Input: part model. Units: mm. Frame: model coordinates. A direction names the side the tool comes from. Give positions to 0.01 mm unless a question says otherwise; leave off trailing zeros. Loops run counter-clockwise (first coordinate to the right, second up) from the corner with the lowest first, then second, coordinate; pieces in that order, holes last.
from build123d import *

# Parameters (mm, degrees)
SKETCH1_R                       = 6.35
SKETCH1_R_2                     = 3.96875
BOSS_EXTRUDE1_DEPTH             = 7.62
SKETCH2_W                       = 4.62
SKETCH2_H                       = 1
F_1_32_0_03125_DIAMETER_HOLE1_D = 0.79375


with BuildPart() as part:
    # Sketch1 → Boss-Extrude1 (new body)
    with BuildSketch(Plane(origin=(0, 0, 0), x_dir=(0, 0, -1), z_dir=(1, 0, 0))):
        with Locations(Location((0, 0, 0), (0, 0, 180))):
            Circle(SKETCH1_R)
        with Locations(Location((0, 0, 0), (0, 0, 180))):
            Circle(SKETCH1_R_2, mode=Mode.SUBTRACT)
    extrude(amount=BOSS_EXTRUDE1_DEPTH)

    # Sketch2 → Cut-Revolve1 (revolve, cut)
    with BuildSketch(Plane.XY, mode=Mode.PRIVATE) as cut_revolve1_sk:
        with Locations((5.31, 5.85)):
            Rectangle(SKETCH2_W, SKETCH2_H)
    revolve(cut_revolve1_sk.sketch.rotate(Axis((7.62, 0, 0), (-1, 0, 0)), 270), axis=Axis((7.62, 0, 0), (-1, 0, 0)), mode=Mode.SUBTRACT)

    # Sketch3 → #60 (0.04) Diameter Hole1 (revolve, cut)
    with BuildSketch(Plane.YZ.offset(1.524)):
        Polygon((0, 0), (0, 25.705237194), (0.508, 25.4), (0.508, 0), align=None)
    revolve(axis=Axis((1.524, 0, -6.35), (0, 0, 1)), mode=Mode.SUBTRACT)

    # 1/32 (0.03125) Diameter Hole1 (through all)
    with Locations(Plane(origin=(0, 0, -5.08), x_dir=(1, 0, 0), z_dir=(0, 0, -1))):
        with Locations((1.524, 5.08)):
            Hole(F_1_32_0_03125_DIAMETER_HOLE1_D / 2)


solid = part.part
(1) Cut plane C-C (x = 6). Return the cut outline in (y, z), and give its area (3 significant figures).
Values follow:
outline: circle Ø10.7 at (0, 0); hole circle Ø7.94 at (0, 0)
area: 40.4 mm2
(2) Cut plane D-D (z = -3.25). Return the cut outline in (x, y), and give its area (3 significant figures).
Values follow:
outline: (0, -5.46) - (1.39, -5.46) arc R0.4 cw (long way) to (1.65, -5.46) - (3, -5.46) - (3, -4.25) - (7.62, -4.25) - (7.62, -2.28) - (0, -2.28) - close; (0, 2.28) - (7.62, 2.28) - (7.62, 4.25) - (3, 4.25) - (3, 5.46) - (0, 5.46) - close
area: 36.8 mm2
(3) Mould query, pull axis Y, two halves, no side actions, for faces 1 (the flat face through (3, -5, 3)), 2 (the cylindrical face through (3.757, 3.874, -0.86)), 3 (the cylindrical face through (5.342, -5.223, -1.16)). Classes: +Y half, -Y half, draft (parallel to the pull), parting line (faces both ways), or undercut.
Values follow:
face 1: draft
face 2: undercut
face 3: parting line
(4) Reachability of faces 4 (the cylindrical face through (1.48, 6.2, -1.38)), 5 (the cylindrical face through (1.02, -0.07, 5.13)) from +Z, -Z, +X, -X, +Y, -Y: full face, straight path, thin tool, end or side. Return the list, or none.
Values follow:
face 4: +X, -X
face 5: +Z
(5) Pin query (flat end, axial travel): pin 1 Ø2 at (x, z) = (7, -2.5) entering from -Y; pin 2 Ø1.5 at (x, z) = (4, -3.5) entering from +Y; pin 3 Ø0.6 at (x, y) = (1.524, 0) entering from +Z. Return the tip coordinate at first contact, or that it passes through.
Values follow:
pin 1: stops at y = -5.14
pin 2: stops at y = 4.59
pin 3: stops at z = -3.96
(6) Cut plane B-B (y = 0). Return the cut outline in (x, z), and give its area (3 significant figures).
Values follow:
outline: (0, -6.35) - (3, -6.35) - (3, -5.35) - (7.62, -5.35) - (7.62, -3.97) - (0, -3.97) - close; (0, 3.97) - (1.02, 3.97) - (1.02, 6.35) - (0, 6.35) - close; (2.03, 3.97) - (7.62, 3.97) - (7.62, 5.35) - (3, 5.35) - (3, 6.35) - (2.03, 6.35) - close
area: 24.6 mm2
(7) Cut plane A-A (z = 0). Return the cut outline in (x, y).
Values follow:
outline: (0, -6.35) - (3, -6.35) - (3, -5.35) - (7.62, -5.35) - (7.62, -3.97) - (0, -3.97) - close; (0, 3.97) - (7.62, 3.97) - (7.62, 5.35) - (3, 5.35) - (3, 6.35) - (0, 6.35) - close; hole circle Ø0.79 at (1.52, -5.08)
(8) Ray query, probe 1 along X at (y, z) = (-5.08, -0.5); probe 2 along Y at (x, z) = (5.75, 0); probe 3 along Z at (x, y) = (0.5, -3). Return the intervals inside material, ascending.
Values follow:
probe 1: x = 0 to 1.13, 1.92 to 7.62
probe 2: y = -5.35 to -3.97, 3.97 to 5.35
probe 3: z = -5.6 to -2.6, 2.6 to 5.6
